Print and shaded views of the part. All mm, measured from the part's lowest x, y and z. A direction names the side the tool comes from. Round coordinates to 2 decimals unless told otherwise and drop trailing zeros. Order: outer loops, then holes, each group sorted by start corner. A loop starts at its lowest first (then second) coordinate and runs counter-clockwise, first axis right, second up. Notation, with made-up numbers: (-25, 26) - (-15, 26) arc R11 cw to (-15, 42) - close; hole circle Ø3 at (0, -38). An arc over 180 degrees is marked (long way). Write item = value, one per line.
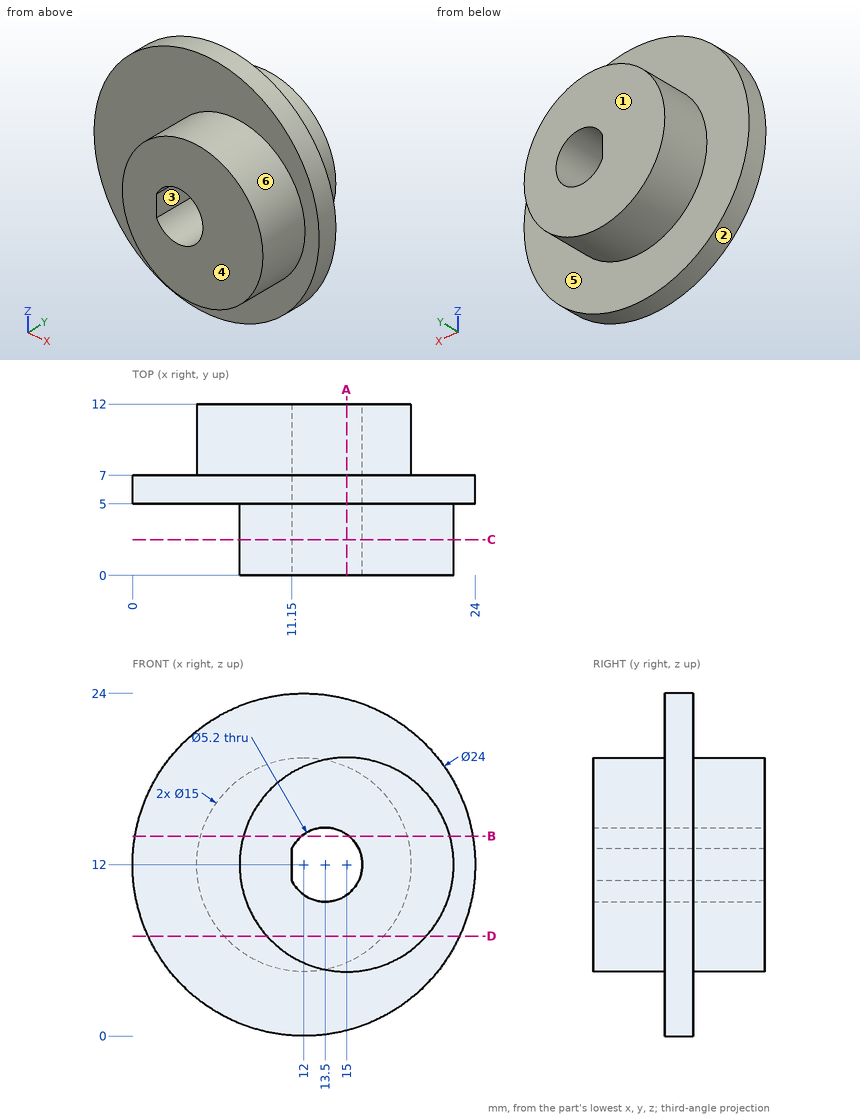
(1) Band-saw the part on A-A on x = 15. List the corners of the cut face in (y, z), plus the area to 3 significant figures.
Solved:
outline = (0, 4.5) - (5, 4.5) - (5, 0.38) - (7, 0.38) - (7, 5.13) - (12, 5.13) - (12, 9.88) - (0, 9.88) - close; (0, 14.12) - (12, 14.12) - (12, 18.87) - (7, 18.87) - (7, 23.62) - (5, 23.62) - (5, 19.5) - (0, 19.5) - close
area = 139 mm²
(2) Drop flat-ended pins along their axis: pin 1 (3 mm diameter, centred on x = 17.5, y = 4, fed in from -Z); pin 2 (3 mm diameter, centred on x = 8, y = 1.5, fed in from +Z); pin 3 (1 mm diameter, centred on x = 8.5, z = 17, fed in from -Y); pin 4 (12 mm diameter, centred on x = 16, z = 3, fed in from -Y). Give the stop position or say it passes through.
Solved:
pin_1 = 0.83
pin_2 = 17.1
pin_3 = 5
pin_4 = 0
(3) Probe line 1 along X through (y, z) = (6.75, 12); line 2 along Y through (x, z) = (12.5, 20.5); line 3 along Y through (x, z) = (6.5, 16.75). List the from-to ranges inside material, lowest first.
Solved:
line_1 = 0 to 11.15, 16.1 to 24
line_2 = 5 to 7
line_3 = 5 to 12
(4) Tool access for the marked faces 4, 5 and 6: list every direction of +Z, -Z, +X, -X, +Y, -Y with a clear straight run to the whole face (end or side of a thin tool).
Solved:
face_4 = +Z, -Z, +X, -X, -Y
face_5 = +Y
face_6 = -Y
(5) Band-saw the part on C-C on y = 2.5. List the corners of the cut face in (x, z).
Solved:
outline = circle Ø15 at (15, 12); hole (11.15, 10.89) arc R2.6 ccw (long way) to (11.15, 13.11) - close
(6) Band-saw the part on D-D on z = 7. List the corners of the cut face in (x, y).
Solved:
outline = (1.09, 5) - (9.41, 5) - (9.41, 0) - (20.59, 0) - (20.59, 5) - (22.91, 5) - (22.91, 7) - (17.59, 7) - (17.59, 12) - (6.41, 12) - (6.41, 7) - (1.09, 7) - close
(7) Pull direction X, two halves, no side cores. Call the marked faces 1, 2 and 3: released by +X, released by -X, zero draft, split by the parting line, or undercut.
Solved:
face_1 = zero draft
face_2 = split by the parting line
face_3 = undercut
(8) Band-saw the part on B-B on z = 14. List the corners of the cut face in (x, y), plus the area to 3 significant figures.
Solved:
outline = (0.17, 5) - (7.77, 5) - (7.77, 0) - (11.84, 0) - (11.84, 12) - (4.77, 12) - (4.77, 7) - (0.17, 7) - close; (15.16, 0) - (22.23, 0) - (22.23, 5) - (23.83, 5) - (23.83, 7) - (19.23, 7) - (19.23, 12) - (15.16, 12) - close
area = 152 mm²
